Build history of the part. All positions in model axes, mm. Coordinates: 2 decimals unless noted, no trailing zeros. Order: outer loops, then holes, each group sorted by start corner. A loop starts at its lowest first (then second) coordinate and runs counter-clockwise, first axis right, second up. Notation, with made-up numbers: (32.25, 47) - (74.25, 47) arc R18 ccw to (74.25, 52) - close; hole circle Ø1 at (-3, 89.25). An arc over 180 degrees is marked (long way). One line per item, written item: value.
from build123d import *

# Parameters (mm, degrees)
SKETCH1_R           = 2.0193
BOSS_EXTRUDE1_DEPTH = 56.515


with BuildPart() as part:
    # Sketch1 → Boss-Extrude1 (new, symmetric)
    with BuildSketch(Plane(origin=(0, 0, 0), x_dir=(0, 0, -1), z_dir=(1, 0, 0))):
        with BuildLine():
            ThreePointArc((6.874999966, 0), (6.860422465, 0.447468582), (6.816751782, 0.893039571))
            Line((6.816751782, 0.893039571), (4.181770846, 5.456960429))
            ThreePointArc((4.181770846, 5.456960429), (3.437499983, 5.953924622), (2.634980936, 6.35))
            Line((2.634980936, 6.35), (-2.634980936, 6.35))
            ThreePointArc((-2.634980936, 6.35), (-3.437499983, 5.953924622), (-4.181770846, 5.456960429))
            Line((-4.181770846, 5.456960429), (-6.816751782, 0.893039571))
            ThreePointArc((-6.816751782, 0.893039571), (-6.874999966, 0), (-6.816751782, -0.893039571))
            Line((-6.816751782, -0.893039571), (-4.181770846, -5.456960429))
            ThreePointArc((-4.181770846, -5.456960429), (-3.437499983, -5.953924622), (-2.634980936, -6.35))
            Line((-2.634980936, -6.35), (2.634980936, -6.35))
            ThreePointArc((2.634980936, -6.35), (3.437499983, -5.953924622), (4.181770846, -5.456960429))
            Line((4.181770846, -5.456960429), (6.816751782, -0.893039571))
            ThreePointArc((6.816751782, -0.893039571), (6.860422465, -0.447468582), (6.874999966, 0))
        make_face()
        with Locations(Location((0, 0, 0), (0, 0, 180))):
            Circle(SKETCH1_R, mode=Mode.SUBTRACT)
    extrude(amount=BOSS_EXTRUDE1_DEPTH, both=True)


solid = part.part
1. Probe line 1 along Y through (x, z) = (2, 0); line 2 along Z through (x, y) = (-37, 0.75); line 3 along Y through (x, z) = (10.5, 1.75). List the from-to ranges inside material, lowest first.
Values found:
line 1: y = -6.35 to -2.02, 2.02 to 6.35
line 2: z = -6.83 to -1.87, 1.87 to 6.83
line 3: y = -6.35 to -1.01, 1.01 to 6.35
2. Band-saw the part on B-B, the plane x = 44. Give the cut face in (y, z) (3 decimals).
Values found:
outline: (-6.35, -2.635) arc R6.875 ccw to (-5.457, -4.182) - (-0.893, -6.817) arc R6.875 ccw to (0.893, -6.817) - (5.457, -4.182) arc R6.875 ccw to (6.35, -2.635) - (6.35, 2.635) arc R6.875 ccw to (5.457, 4.182) - (0.893, 6.817) arc R6.875 ccw to (-0.893, 6.817) - (-5.457, 4.182) arc R6.875 ccw to (-6.35, 2.635) - close; hole circle Ø4.039 at (0, 0)
3. Band-saw the part on A-A, the plane z = 0. Give the cut face in (x, y) (3 decimals), and give its area (3 significant figures).
Values found:
outline: (-56.515, -6.35) - (56.515, -6.35) - (56.515, -2.019) - (-56.515, -2.019) - close; (-56.515, 2.019) - (56.515, 2.019) - (56.515, 6.35) - (-56.515, 6.35) - close
area: 979 mm2
4. Flat gauge pins, fed straight in: P1, Ø2, axis at x = 39, y = -2, coming from the -Z side (3 decimals); P2, Ø4, axis at x = -33, z = -3.5, coming from the +Y side. Where does each tip first touch, or does it go through?
Values found:
P1: stops at z = -6.755
P2: stops at y = 6.35
5. Two-plate mould, pull along Y, no slides. Class faces 1 (the face through (-0.791, -0.607, 1.926)), 2 (the face through (0.79, 3.14, -5.52)), 3 (the face through (0.79, -3.21, -5.48)), 4 (the face through (0.791, 0.013, 6.875)): pulls with the +Y half, pulls with the -Y half, needs draft (parallel to the pull), parting line crosses it, or undercut.
Values found:
face 1: undercut
face 2: pulls with the +Y half
face 3: pulls with the -Y half
face 4: parting line crosses it
6. Band-saw the part on D-D, the plane z = -5.25. Give the cut face in (x, y) (3 decimals), and give its area (3 significant figures).
Values found:
outline: (-56.515, -3.607) - (56.515, -3.607) - (56.515, 3.607) - (-56.515, 3.607) - close
area: 815 mm2
7. Band-saw the part on C-C, the plane y = 3.25. Give the cut face in (x, z) (3 decimals), and give its area (3 significant figures).
Values found:
outline: (-56.515, -5.456) - (56.515, -5.456) - (56.515, 5.456) - (-56.515, 5.456) - close
area: 1,230 mm2
